Could you check a few things on this model? Use its own coordinates, in mm. A direction names the side the tool comes from. Round coordinates to 2 decimals unless told otherwise and drop trailing zeros. Loops run counter-clockwise (first coordinate to the right, second up) from the corner with the lowest first, then second, coordinate; pieces in that order, holes last. Notation, with made-up numbers: M -24,58.25 L 13,58.25 A16 ccw 13,82.25 Z; hole C 13.5,-14 d2. An arc over 180 degrees is marked long. One line per item, written item: value. Start each with the question number.
Q1. Imagine slicing it at B-B (x = -13.5). Please give me the cut outline in (y, z), then the cut area to 3 significant figures.
Q2. Imagine slicing it at A-A (x = -67). Please give me the cut outline in (y, z), then the cut area to 3 significant figures.
Q3. Thinking about a two-plate mould opening in X: for faces 4 (the face through (-68, 9, 5)), 5 (the face through (-4.77, 5, 74)), 6 (the face through (-67.7, 0.8, 86.7)), 7 (the face through (2.54, 2.36, 71.9)), which applies, released by +X, released by -X, zero draft, split by the parting line, or undercut?
Q4. Please list where these lines run through material, in increasing order: line 1 along X through (y, z) = (0.8, 88); line 2 along Z through (x, y) = (-3, 0.85); line 3 along X through (y, z) = (13.75, 12).
Q5. Imagine slicing it at C-C (y = 8.5). Please give me the cut outline in (x, z).
Q6. I'm going to push flat-ended pins straight in: pin 1 Ø2 at (y, z) = (14.5, 18.5) entering from -X; pin 2 Ø3 at (x, y) = (-12.5, 4) entering from -Z; pin 3 Ø3 at (x, z) = (-3, 88) entering from +Y; pin 4 Ø2.5 at (y, z) = (4, 15.5) entering from +X. Where does each tip first touch, or does it pass through?
Q7. Which directions (+Z, -Z, +X, -X, +Y, -Y) give clear straight access to the entire face, cutting with the end or side of a thin tool? Please do faces 1 (the face through (-1, 5, 77)), 2 (the face through (-15, 7.5, 14)), 3 (the face through (-55, 9, 5)).
Q8. Imagine slicing it at D-D (z = 82). Please give me the cut outline in (x, y), then the cut area to 3 significant figures.
Autodesk Inventor part; units mm, degrees
ref_plane "YZ Plane" through (0, 0, 0) normal (1, 0, 0) x (0, 1, 0)
ref_plane "XZ Plane" through (0, 0, 0) normal (0, 1, 0) x (-1, 0, 0)
ref_plane "XY Plane" through (0, 0, 0) normal (0, 0, 1) x (1, 0, 0)
sketch "Эскиз1" plane through (0, 0, 0) normal (0, 1, 0) x (-1, 0, 0)
  line L0 (0, 0) -> (70, 0)
  line L1 (70, 0) -> (70, 90)
  line L2 (70, 90) -> (0, 90)
  line L3 (0, 90) -> (0, 0)
  dimension "d0" = 70
  dimension "d1" = 90
extrude "Выдавливание1" add sketch "Эскиз1" along normal blind 1.5
fillet "Сопряжение1" radius 1 4 edges at (0, 0.75, 90) (0, 0.75, 0) (-70, 0.75, 90) (-70, 0.75, 0)
sketch "Эскиз2" plane through (0, 1.5, 0) normal (0, 1, 0) x (1, 0, 0)
  line L0 (-59.5, -74) -> (-73.5, -74)
  line L1 (-73.5, -74) -> (-73.5, -65)
  line L2 (-73.5, -65) -> (-59.5, -65)
  line L3 (-59.5, -65) -> (-59.5, -74)
  line L4 (-69, -90) -> (-1, -90)
  line L5 (-70, -1) -> (-70, -89)
  point P0 (0, 0)
  dimension "d5" = 16
  dimension "d6" = 9
  dimension "d7" = 14
  dimension "d8" = 3.5
extrude "Выдавливание2" add sketch "Эскиз2" along normal blind 11
sketch "Эскиз3" plane through (0, 1.5, 0) normal (0, 1, 0) x (1, 0, 0)
  line L0 (5, -77) -> (-4.77, -77)
  line L1 (-4.77, -77) -> (-4.77, -71)
  line L2 (-4.77, -71) -> (5, -71)
  line L3 (5, -71) -> (5, -77)
  line L4 (-69, -90) -> (-1, -90)
  line L5 (0, -89) -> (0, -1)
  point P0 (0, 0)
  dimension "d11" = 6
  dimension "d12" = 13
  dimension "d13" = 5
extrude "Выдавливание3" add sketch "Эскиз3" along normal blind 8
fillet "Сопряжение2" radius 3 4 edges at (0.115, 9.5, 71) (0.115, 9.5, 77) (2.5, 1.5, 77) (2.5, 1.5, 71)
sketch "Эскиз4" plane through (0, 1.5, 0) normal (0, 1, 0) x (1, 0, 0)
  line L0 (-20, -17) -> (-36, -17)
  line L1 (-36, -17) -> (-36, 4)
  line L2 (-36, 4) -> (-20, 4)
  line L3 (-20, 4) -> (-20, -17)
  line L4 (-1, 0) -> (-69, 0)
  line L5 (0, -71) -> (0, -1)
  point P0 (0, 0)
  dimension "d17" = 21
  dimension "d18" = 16
  dimension "d19" = 4
  dimension "d20" = 20
extrude "Выдавливание4" add sketch "Эскиз4" along normal blind 13
sketch "Эскиз5" plane through (0, 1.5, 0) normal (0, 1, 0) x (1, 0, 0)
  line L0 (-55, -14) -> (-68, -14)
  line L1 (-68, -14) -> (-68, 4)
  line L2 (-68, 4) -> (-55, 4)
  line L3 (-55, 4) -> (-55, -14)
  line L4 (-70, -1) -> (-70, -65)
  line L5 (-36, 0) -> (-69, 0)
  point P0 (0, 0)
  dimension "d27" = 16
  dimension "d23" = 18
  dimension "d24" = 13
  dimension "d25" = 2
  dimension "d26" = 4
extrude "Выдавливание5" add sketch "Эскиз5" along normal blind 16
sketch "Эскиз6" plane through (0, 1.5, 0) normal (0, 1, 0) x (1, 0, 0)
  arc A0 (-1, -90) -> (0, -89) centre (-1, -89) ccw
  arc A1 (-70, -89) -> (-69, -90) centre (-69, -89) ccw
  circle A2 centre (-67, -87.4129) radius 1
  line L0 (-68, -14) -> (-68, 0)
  line L1 (-68, 0) -> (-69, 0)
  arc A3 (-69, 0) -> (-70, -1) centre (-69, -1) ccw
  line L2 (-70, -1) -> (-70, -65)
  line L3 (-70, -65) -> (-59.5, -65)
  line L4 (-59.5, -65) -> (-59.5, -74)
  line L5 (-59.5, -74) -> (-70, -74)
  line L6 (-70, -74) -> (-70, -89)
  arc A4 (-70, -89) -> (-69, -90) centre (-69, -89) ccw
  line L7 (-69, -90) -> (-1, -90)
  arc A5 (-1, -90) -> (0, -89) centre (-1, -89) ccw
  line L8 (0, -89) -> (0, -77)
  line L9 (0, -77) -> (-4.77, -77)
  line L10 (-4.77, -77) -> (-4.77, -71)
  line L11 (-4.77, -71) -> (0, -71)
  line L12 (0, -71) -> (0, -1)
  arc A6 (0, -1) -> (-1, 0) centre (-1, -1) ccw
  line L13 (-1, 0) -> (-20, 0)
  line L14 (-20, 0) -> (-20, -17)
  line L15 (-20, -17) -> (-36, -17)
  line L16 (-36, -17) -> (-36, 0)
  line L17 (-36, 0) -> (-55, 0)
  line L18 (-55, 0) -> (-55, -14)
  line L19 (-55, -14) -> (-68, -14)
  circle A7 centre (-3, -88) radius 1
  point P0 (0, 0)
  dimension "d29" = 2
  dimension "d30" = 2
  dimension "d31" = 64
  dimension "d32" = 70
  dimension "d33" = 3
extrude "Выдавливание6" cut sketch "Эскиз6" against normal blind 3 contours A2 | A7
sketch "Эскиз7" plane through (0, 1.5, 0) normal (0, 1, 0) x (1, 0, 0)
  line L0 (-36, -17) -> (-20, -17)
  line L1 (-20, 0) -> (-20, -17)
  line L2 (-20, -17) -> (-9, -17)
  line L3 (-9, -17) -> (-9, -12)
  line L4 (-9, -12) -> (-20, -12)
  line L5 (-20, -12) -> (-20, -17)
  point P0 (0, 0)
  dimension "d36" = 11
  dimension "d37" = 5
extrude "Выдавливание7" add sketch "Эскиз7" along normal blind 6
equation "\"d34\" = d33"
properties part number "Stemboard"
Report:
1. outline: M 0,0 L 1.5,0 L 1.5,12 L 7.5,12 L 7.5,17 L 1.5,17 L 1.5,90 L 0,90 Z
1. area: 165 mm²
2. outline: M 0,0 L 1.5,0 L 1.5,-4 L 17.5,-4 L 17.5,14 L 1.5,14 L 1.5,65 L 12.5,65 L 12.5,74 L 1.5,74 L 1.5,86.41 L 0,86.41 Z; M 0,88.41 L 1.5,88.41 L 1.5,90 L 0,90 Z
2. area: 519 mm²
3. face 4: released by -X
3. face 5: undercut
3. face 6: undercut
3. face 7: zero draft
4. line 1: x = -70 to -67.81, -66.19 to -4, -2 to 0
4. line 2: z = 0 to 87, 89 to 90
4. line 3: x = -68 to -55, -36 to -20
5. outline: M -73.5,65 L -59.5,65 L -59.5,74 L -73.5,74 Z; M -68,-4 L -55,-4 L -55,14 L -68,14 Z; M -36,-4 L -20,-4 L -20,17 L -36,17 Z; M -4.77,71.76 L 5,71.76 L 5,76.24 L -4.77,76.24 Z
6. pin 1: passes through
6. pin 2: stops at z = 12
6. pin 3: stops at y = 1.5
6. pin 4: stops at x = -9
7. face 1: +Z, +X, -X, +Y
7. face 2: +Z, -Z, +X, +Y
7. face 3: +Z, -Z, +Y
8. outline: M -70,0 L 0,0 L 0,1.5 L -70,1.5 Z
8. area: 105 mm²
